The model under review builds one solid part; all positions refer to its coordinate system, in mm. Face numbers are marked on the shaded views. Coordinates: 2 decimals unless noted, no trailing zeros. Order: outer loops, then holes, each group sorted by start corner. A loop starts at its lowest first (then second) coordinate and runs counter-clockwise, first axis right, second up. Notation, with made-up numbers: (1.25, 17.5) - (8.25, 17.5) arc R5 ccw to (8.25, 22.5) - close; hole circle Ø1 at (79.5, 42.5). An arc over 180 degrees is marked (long way). Answer in a Markdown table with one row per item.
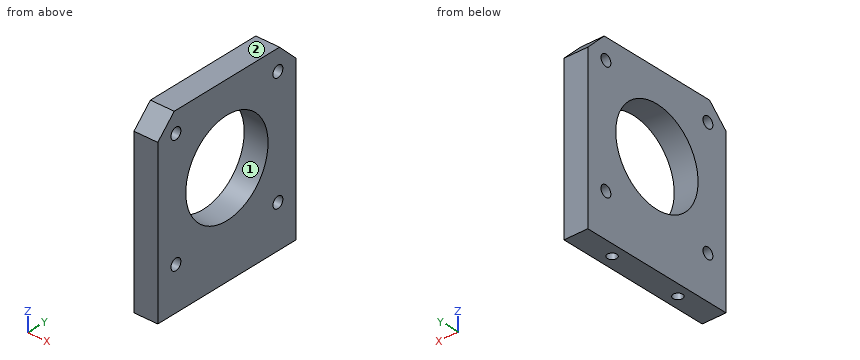
```python
from build123d import *

# Parameters (mm, degrees)
SKETCH_R             = 12.5
SKETCH_R_2           = 1.5
PAD_DEPTH            = 6.35
SKETCH011_R          = 1.25
HOLE_DEPTH           = 15
HOLE_TIPS_R          = 1.25
BODY_PLACEMENT_ANGLE = 0.285111


with BuildPart() as part:
    # Sketch → Pad (new body)
    with BuildSketch(Plane.YZ):
        Polygon((-21, -27), (21, -27), (21, 16), (16, 21), (-16, 21), (-21, 16), align=None)
        Circle(SKETCH_R, mode=Mode.SUBTRACT)
        with Locations((15.495, 15.495)):
            Circle(SKETCH_R_2, mode=Mode.SUBTRACT)
        with Locations((15.495, -15.495)):
            Circle(SKETCH_R_2, mode=Mode.SUBTRACT)
        with Locations((-15.495, -15.495)):
            Circle(SKETCH_R_2, mode=Mode.SUBTRACT)
        with Locations((-15.495, 15.495)):
            Circle(SKETCH_R_2, mode=Mode.SUBTRACT)
    extrude(amount=PAD_DEPTH)

    # Sketch011 (on Face4 of Pad) → Hole (cut)
    with BuildSketch(Plane(origin=(0, 0, -27), x_dir=(1, 0, 0), z_dir=(0, 0, -1))):
        with Locations((3.175, 10)):
            Circle(SKETCH011_R)
        with Locations((3.175, -10)):
            Circle(SKETCH011_R)
    extrude(amount=-HOLE_DEPTH, mode=Mode.SUBTRACT)

    # Hole tips → Hole tip 1 section 0
    with BuildSketch(Plane(origin=(0, 0, -12), x_dir=(1, 0, 0), z_dir=(0, 0, -1)), mode=Mode.PRIVATE) as hole_tip_1_s0:
        with Locations((3.175, 10)):
            Circle(HOLE_TIPS_R)
    loft([hole_tip_1_s0.sketch, Vertex(3.175, -10, -11.248924)], mode=Mode.SUBTRACT)

    # Hole tips → Hole tip 2 section 0
    with BuildSketch(Plane(origin=(0, 0, -12), x_dir=(1, 0, 0), z_dir=(0, 0, -1)), mode=Mode.PRIVATE) as hole_tip_2_s0:
        with Locations((3.175, -10)):
            Circle(HOLE_TIPS_R)
    loft([hole_tip_2_s0.sketch, Vertex(3.175, 10, -11.248924)], mode=Mode.SUBTRACT)


with BuildPart() as part_1:
    # Body placement: moved
    add(part.part.moved(Location((89.750311, 49.797284, 37.128014))).rotate(Axis((89.750311, 49.797284, 37.128014), (0, 0, 1)), BODY_PLACEMENT_ANGLE))


solid = part_1.part
```
Item 1: To check wall thickness, follow line 1 (Z direction, x = 91.5, y = 34); line 2 (Z direction, x = 92, y = 35.5); line 3 (Y direction, x = 90.75, z = 18.5). State the ranges of each line that lie inside material, in increasing order. Write a range as from..to.
Check values:
| item | result |
|---|---|
| line 1 | 10.13..20.17, 23.1..51.16, 54.09..58.13 |
| line 2 | 10.13..20.72, 22.55..51.71, 53.54..58.13 |
| line 3 | 28.8..70.8 |
Item 2: Clearance check with a flat-ended pin moving along its axis: pin 1 Ø1 at (y, z) = (61, 50) entering from -X. State where the tip first meets the part, or that it passes through.
Check values:
| item | result |
|---|---|
| pin 1 | x = 89.69 |
Item 3: We need section A-A, the plane z = 36. Write out the cut boundary in (x, y).
Check values:
| item | result |
|---|---|
| outline | (89.65, 70.8) - (89.69, 62.25) - (96.04, 62.28) - (96, 70.83) - close; (89.81, 37.35) - (89.85, 28.8) - (96.2, 28.83) - (96.16, 37.38) - close |
Item 4: We need section B-B, the plane y = 34.5. State how many separate pieces and enclosed holes the cut face has, then the cut area to 3 significant figures.
Check values:
| item | result |
|---|---|
| separate pieces | 3 |
| enclosed holes | 0 |
| area | 267 mm^2 |
Item 5: We need section C-C, the plane z = 19.5. Write out the cut boundary in (x, y), then the cut area to 3 significant figures.
Check values:
| item | result |
|---|---|
| outline | (89.65, 70.8) - (89.85, 28.8) - (96.2, 28.83) - (96, 70.83) - close; hole circle Ø2.5 at (92.88, 59.81); hole circle Ø2.5 at (92.98, 39.81) |
| area | 257 mm^2 |
Item 6: Mouldability with a two-part tool opening along Y and no side actions: class the marked faces 1 and 2 as +Y half, -Y half, draft (parallel to the pull), parting line (faces both ways), or undercut.
Check values:
| item | result |
|---|---|
| face 1 | undercut |
| face 2 | draft |
